Autodesk Inventor part; units mm, degrees
ref_plane "YZ Plane" through (0, 0, 0) normal (1, 0, 0) x (0, 1, 0)
ref_plane "XZ Plane" through (0, 0, 0) normal (0, 1, 0) x (-1, 0, 0)
ref_plane "XY Plane" through (0, 0, 0) normal (0, 0, 1) x (1, 0, 0)
sketch "Sketch1" plane through (0, 0, 0) normal (1, 0, 0) x (0, 1, 0)
  line L0 (0, 0) -> (-25.4, 0)
  line L1 (-25.4, 0) -> (-25.4, -25.4)
  line L2 (-25.4, -25.4) -> (0, -25.4)
  line L3 (0, -25.4) -> (0, 0)
  dimension "d0" = 25.4
  dimension "d1" = 25.4
extrude "Extrusion1" add sketch "Sketch1" along normal blind 3.175
sketch "Sketch2" plane through (3.175, 0, 0) normal (1, 0, 0) x (0, 0, -1)
  line L0 (0, 0) -> (3.175, 0)
  line L1 (3.175, 0) -> (3.175, -25.4)
  line L2 (3.175, -25.4) -> (0, -25.4)
  line L3 (0, -25.4) -> (0, 0)
  dimension "d4" = 3.175
  dimension "d5" = 25.4
extrude "Extrusion2" add sketch "Sketch2" along normal blind 47.625
sketch "Sketch3" plane through (3.175, -25.4, -3.175) normal (0, 0, -1) x (-1, 0, 0)
  line L0 (-47.625, 0) -> (-47.625, 25.4)
  line L1 (0, 0) -> (0, 25.4)
  line L2 (0, 0) -> (-47.625, 0)
  point P0 (3.175, 25.4)
  point P1 (-31.75, 12.7)
  point P2 (-15.875, 12.7)
  dimension "d8" = 15.875
  dimension "d9" = 15.875
  dimension "d10" = 15.875
  dimension "d11" = 12.7
hole "Hole1" at (34.925, -12.7, -3.175) at (19.05, -12.7, -3.175) direction (0, 0, 1) diameter 6.35 end through all
sketch "Sketch4" plane through (3.175, 0, 0) normal (1, 0, 0) x (0, 0, -1)
  line L0 (25.4, 0) -> (3.175, 0)
  line L1 (25.4, -25.4) -> (25.4, 0)
  point P0 (0, 0)
  point P1 (12.7, -12.7)
  dimension "d19" = 12.7
  dimension "d20" = 12.7
hole "Hole2" at (3.175, -12.7, -12.7) direction (-1, 0, 0) diameter 6.35 end through all
fillet "Fillet1" radius 2.54 1 edges at (50.8, -12.7, -3.175)
fillet "Fillet2" radius 2.54 1 edges at (3.175, -12.7, -3.175)
fillet "Fillet3" radius 2.54 1 edges at (3.175, -12.7, -25.4)
properties part number "L bracket"
The listing builds one solid part. Answer for the finished solid, in the listing's coordinates (mm). A direction names the side the tool comes from. Round coordinates to 2 decimals unless told otherwise and drop trailing zeros. Loops run counter-clockwise (first coordinate to the right, second up) from the corner with the lowest first, then second, coordinate; pieces in that order, holes last.
1) For faces 5 (the face through (27, -13, -3.175)), 6 (the face through (18.1, -9.67, -1.57)), determine the directions among +Z, -Z, +X, -X, +Y, -Y from which every point of the face is accessible in a straight line to the end or side of a thin tool.
Outcome:
face 5: -Z, +X, +Y, -Y
face 6: +Z, -Z
2) A cutting plane is placed at D-D on y = -19. Determine the outline of the cut face in (x, z) (3 decimals).
Outcome:
outline: (0, -25.4) - (0.635, -25.4) arc R2.54 ccw to (3.175, -22.86) - (3.175, -5.715) arc R2.54 cw to (5.715, -3.175) - (48.26, -3.175) arc R2.54 ccw to (50.8, -0.635) - (50.8, 0) - (0, 0) - close
3) Consider line 1 (Y direction, x = 1.05, z = -12.7) (3 decimals); line 2 (Z direction, x = 37, y = -18.75) (3 decimals); line 3 (Z direction, x = 1.4, y = -12.7) (3 decimals). Determine where each line is inside the solid, lowest interval first.
Outcome:
line 1: y = -25.4 to -15.875, -9.525 to 0
line 2: z = -3.175 to 0
line 3: z = -25.282 to -15.875, -9.525 to 0
4) Given P1, Ø7.5, axis at x = 19, y = -18.5, coming from the -Z side (3 decimals); P2, Ø5, axis at y = -12, z = -6, coming from the +X side; P3, Ø6, axis at y = -7.5, z = -18.5, coming from the +X side (3 decimals); P4, Ø4, axis at x = 34.925, y = -12.7, coming from the +Z side, each flat-ended and moving along its own axis, determine where each tip first touches the part or whether it passes through.
Outcome:
P1: stops at z = -3.175
P2: stops at x = 4.47
P3: stops at x = 3.175
P4: passes through
5) A cutting plane is placed at C-C on z = -12.7. Determine the outline of the cut face in (x, y) (3 decimals).
Outcome:
outline: (0, -25.4) - (3.175, -25.4) - (3.175, -15.875) - (0, -15.875) - close; (0, -9.525) - (3.175, -9.525) - (3.175, 0) - (0, 0) - close
6) For a pull along Z with two mould halves and no side action, classify faces 1 (the face through (1.57, -10.77, -10.18)), 2 (the face through (3.175, -12.9, -16.1)), 3 (the face through (25, -13, 0)), 4 (the face through (2, -13, -25)) as released by +Z, released by -Z, zero draft, split by the parting line, or undercut.
Outcome:
face 1: undercut
face 2: zero draft
face 3: released by +Z
face 4: released by -Z
7) A cutting plane is placed at A-A on y = -12.7. Determine the outline of the cut face in (x, z) (3 decimals).
Outcome:
outline: (0, -25.4) - (0.635, -25.4) arc R2.54 ccw to (3.175, -22.86) - (3.175, -15.875) - (0, -15.875) - close; (0, -9.525) - (3.175, -9.525) - (3.175, -5.715) arc R2.54 cw to (5.715, -3.175) - (15.875, -3.175) - (15.875, 0) - (0, 0) - close; (22.225, -3.175) - (31.75, -3.175) - (31.75, 0) - (22.225, 0) - close; (38.1, -3.175) - (48.26, -3.175) arc R2.54 ccw to (50.8, -0.635) - (50.8, 0) - (38.1, 0) - close
8) A cutting plane is placed at B-B on x = 19.05. Determine the outline of the cut face in (y, z) (3 decimals).
Outcome:
outline: (-25.4, -3.175) - (-15.875, -3.175) - (-15.875, 0) - (-25.4, 0) - close; (-9.525, -3.175) - (0, -3.175) - (0, 0) - (-9.525, 0) - close
